```python
from build123d import *

# Parameters (mm, degrees)
SKETCH_1_W          = 34
SKETCH_1_H          = 30
SKETCH_1_R          = 5.25
EXTRUDE_1_DEPTH     = 30
SKETCH_2_R          = 1.75
CUT_EXTRUDE_1_DEPTH = 10
SKETCH_4_R          = 2
CUT_EXTRUDE_3_DEPTH = 10
SKETCH_5_R          = 1.5
CUT_EXTRUDE_4_DEPTH = 5


with BuildPart() as part:
    # 草图1 → 凸台-拉伸1 (new body)
    with BuildSketch(Plane.XY):
        Rectangle(SKETCH_1_W, SKETCH_1_H)
        Circle(SKETCH_1_R, mode=Mode.SUBTRACT)
    extrude(amount=EXTRUDE_1_DEPTH)

    # 草图2 → 切除-拉伸1 (cut)
    with BuildSketch(Plane.XY.offset(30)):
        with Locations((-8, 0)):
            Circle(SKETCH_2_R)
        with Locations((0, 8)):
            Circle(SKETCH_2_R)
        with Locations((8, 0)):
            Circle(SKETCH_2_R)
        with Locations((0, -8)):
            Circle(SKETCH_2_R)
    extrude(amount=-CUT_EXTRUDE_1_DEPTH, mode=Mode.SUBTRACT)

    # 草图4 → 切除-拉伸3 (cut)
    with BuildSketch(Plane(origin=(0, 15, 0), x_dir=(1, 0, 0), z_dir=(0, 1, 0))):
        with Locations(Location((12, -25, 0), (0, 0, 180))):
            Circle(SKETCH_4_R)
        with Locations(Location((-12, -25, 0), (0, 0, 180))):
            Circle(SKETCH_4_R)
        with Locations(Location((-12, -5, 0), (0, 0, 180))):
            Circle(SKETCH_4_R)
        with Locations(Location((12, -5, 0), (0, 0, 180))):
            Circle(SKETCH_4_R)
    extrude(amount=-CUT_EXTRUDE_3_DEPTH, mode=Mode.SUBTRACT)

    # 草图5 → 切除-拉伸4 (cut)
    with BuildSketch(Plane(origin=(0, -15, 0), x_dir=(-1, 0, 0), z_dir=(0, -1, 0))):
        with Locations(Location((1, -25, 0), (0, 0, 180))):
            Circle(SKETCH_5_R)
        with Locations(Location((6, -25, 0), (0, 0, 180))):
            Circle(SKETCH_5_R)
    extrude(amount=-CUT_EXTRUDE_4_DEPTH, mode=Mode.SUBTRACT)


solid = part.part
```
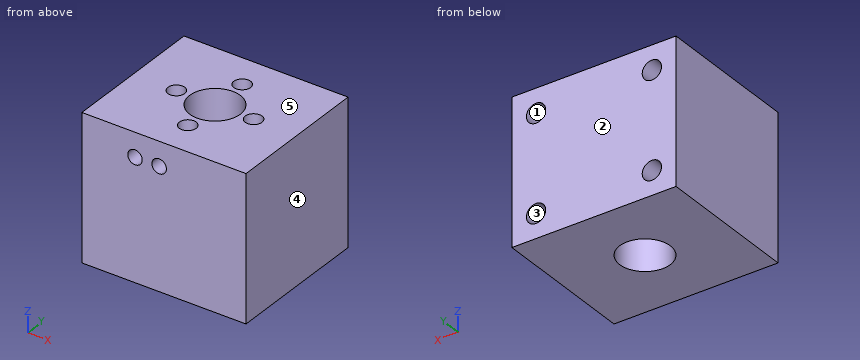
Design review of the part built by this model. Coordinates are the model's own, in mm. Face numbers are marked on the shaded views. A direction names the side the tool comes from. Coordinates: 2 decimals unless noted, no trailing zeros. Order: outer loops, then holes, each group sorted by start corner. A loop starts at its lowest first (then second) coordinate and runs counter-clockwise, first axis right, second up.
1) For the marked faces 1 and 2, list the 3-axis set-ups (+Z, -Z, +X, -X, +Y, -Y) from which the entire face can be reached by the end or side of a thin tool; tool diameter is ignored.
2) Mouldability with a two-part tool opening along X and no side actions: class the marked faces 3, 4 and 5 as +X half, -X half, draft (parallel to the pull), parting line (faces both ways), or undercut.
3) Wall thickness on line 1 along Z through (x, y) = (-12, 10.75); line 2 along Y through (x, z) = (0, 22); line 3 along Z through (x, y) = (-6, -12.9): over which ranges is each line inside the solid? List them lowest first.
4) Take a section at C-C, the plane z = 20.5. Give the boundary of the cut face in (x, y), and give its area (3 significant figures).
5) Clearance check with flat-ended pins moving along their axes: pin 1 (2.5 mm diameter, centred on x = -1, z = 25, fed in from -Y); pin 2 (1.2 mm diameter, centred on x = -11, z = 5.5, fed in from +Y); pin 3 (1 mm diameter, centred on x = 8.5, y = -0.5, fed in from +Z). State where each tip first meets the part, or that it passes through.
6) Take a section at D-D, the plane y = 8. Give the boundary of the cut face in (x, z), and give its area (3 significant figures).
7) Take a section at A-A, the plane y = 0. Give the boundary of the cut face in (x, z), and give its area (3 significant figures).
8) Take a section at B-B, the plane z = 5. Give the boundary of the cut face in (x, y), and give its area (3 significant figures).
Returned:
1. face 1: +Y
1. face 2: +Z, -Z, +X, -X, +Y
2. face 3: undercut
2. face 4: +X half
2. face 5: draft
3. line 1: z = 0 to 3, 7 to 23, 27 to 30
3. line 2: y = -15 to -9.75, -6.25 to -5.25, 5.25 to 6.25, 9.75 to 15
3. line 3: z = 0 to 23.5, 26.5 to 30
4. outline: (-17, -15) - (17, -15) - (17, 15) - (-17, 15) - close; hole circle Ø3.5 at (-8, 0); hole circle Ø10.5 at (0, 0); hole circle Ø3.5 at (0, -8); hole circle Ø3.5 at (0, 8); hole circle Ø3.5 at (8, 0)
4. area: 895 mm2
5. pin 1: stops at y = -10
5. pin 2: stops at y = 5
5. pin 3: stops at z = 20
6. outline: (-17, 0) - (17, 0) - (17, 30) - (1.75, 30) - (1.75, 20) - (-1.75, 20) - (-1.75, 30) - (-17, 30) - close; hole circle Ø4 at (-12, 5); hole circle Ø4 at (-12, 25); hole circle Ø4 at (12, 5); hole circle Ø4 at (12, 25)
6. area: 935 mm2
7. outline: (-17, 0) - (-5.25, 0) - (-5.25, 30) - (-6.25, 30) - (-6.25, 20) - (-9.75, 20) - (-9.75, 30) - (-17, 30) - close; (5.25, 0) - (17, 0) - (17, 30) - (9.75, 30) - (9.75, 20) - (6.25, 20) - (6.25, 30) - (5.25, 30) - close
7. area: 635 mm2
8. outline: (-17, -15) - (17, -15) - (17, 15) - (14, 15) - (14, 5) - (10, 5) - (10, 15) - (-10, 15) - (-10, 5) - (-14, 5) - (-14, 15) - (-17, 15) - close; hole circle Ø10.5 at (0, 0)
8. area: 853 mm2
